Geometry check sheet. Reference: drawing and pictorial views, mm from the part's lowest x, y, z. Give positions to 0.01 mm unless a question says otherwise; leave off trailing zeros. Write each loop counter-clockwise with the first axis right and the second up, starting at its lowest first coordinate (ties: lowest second). Pieces come first, ordered by that corner, then holes. Notation, with made-up numbers: M -33,36.25 L 3,36.25 A29 ccw 3,60.25 Z; hole C -27,3.25 d8. An arc over 180 degrees is marked long. One line per item, written item: value. Start each with the question number.
1. Scan lines: line 1 (X direction, y = 15.5, z = 2.25) (1 decimal); line 2 (X direction, y = 26, z = 9) (1 decimal); line 3 (Y direction, x = 137.5, z = 9) (1 decimal). Record each from-to range of solid material in increasing order.
2. Cross-section at A-A on y = 23.5. Record the cut outline in (x, z).
3. Cross-section at B-B on x = 261. Record the cut outline in (y, z).
4. Cross-section at C-C on z = 3.75. Record the cut outline in (x, y), then the cut area to 3 significant figures.
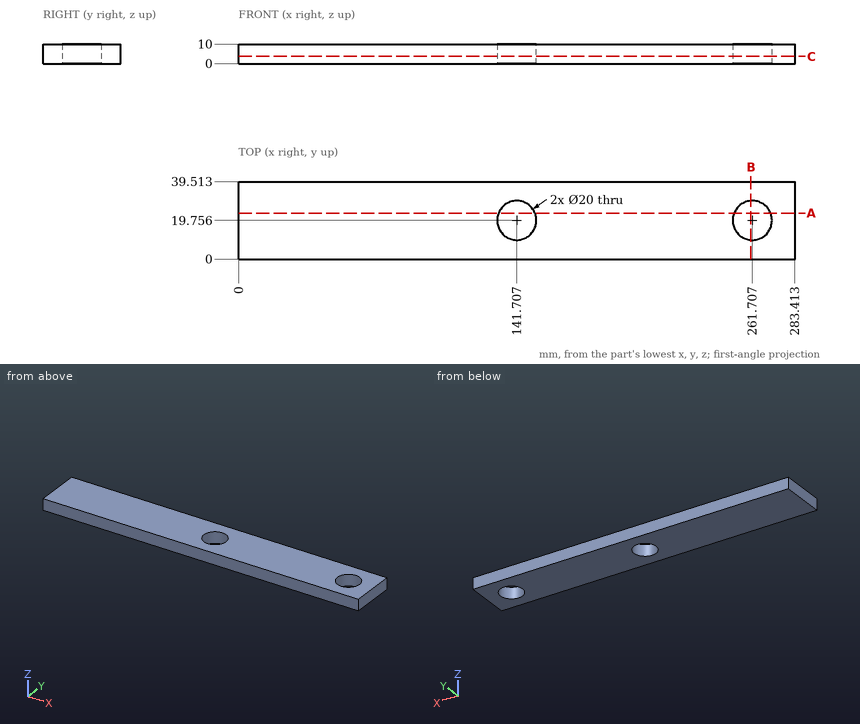
Report:
1. line 1: x = 0 to 132.7, 150.8 to 252.7, 270.8 to 283.4
1. line 2: x = 0 to 133.9, 149.5 to 253.9, 269.5 to 283.4
1. line 3: y = 0 to 10.7, 28.8 to 39.5
2. outline: M 0,0 L 132.43,0 L 132.43,10 L 0,10 Z; M 150.98,0 L 252.43,0 L 252.43,10 L 150.98,10 Z; M 270.98,0 L 283.41,0 L 283.41,10 L 270.98,10 Z
3. outline: M 0,0 L 9.78,0 L 9.78,10 L 0,10 Z; M 29.73,0 L 39.51,0 L 39.51,10 L 29.73,10 Z
4. outline: M 0,0 L 283.41,0 L 283.41,39.51 L 0,39.51 Z; hole C 141.71,19.76 d20; hole C 261.71,19.76 d20
4. area: 10,600 mm^2
